from build123d import *

# Parameters (mm, degrees)
SKETCH1_W               = 210
SKETCH1_H               = 80
SKETCH1_R               = 1.5
SKETCH1_R_2             = 9.5
SKETCH1_W_2             = 20
SKETCH1_H_2             = 20
BOSS_EXTRUDE1_DEPTH     = 3
FILLET1_R               = 5
F_1_4_20_TAPPED_HOLE1_D = 5.1054


with BuildPart() as part:
    # Sketch1 → Boss-Extrude1 (new body)
    with BuildSketch(Plane(origin=(0, 0, 0), x_dir=(1, 0, 0), z_dir=(0, 1, 0))):
        with Locations((105, 40)):
            Rectangle(SKETCH1_W, SKETCH1_H)
        with Locations(Location((52.5, 52.5, 0), (0, 0, 270))):
            Circle(SKETCH1_R, mode=Mode.SUBTRACT)
        with Locations(Location((65, 40, 0), (0, 0, 270))):
            Circle(SKETCH1_R, mode=Mode.SUBTRACT)
        with Locations(Location((52.5, 27.5, 0), (0, 0, 270))):
            Circle(SKETCH1_R, mode=Mode.SUBTRACT)
        with Locations(Location((40, 40, 0), (0, 0, 270))):
            Circle(SKETCH1_R, mode=Mode.SUBTRACT)
        with Locations(Location((157.5, 52.5, 0), (0, 0, 270))):
            Circle(SKETCH1_R, mode=Mode.SUBTRACT)
        with Locations(Location((170, 40, 0), (0, 0, 270))):
            Circle(SKETCH1_R, mode=Mode.SUBTRACT)
        with Locations(Location((157.5, 27.5, 0), (0, 0, 270))):
            Circle(SKETCH1_R, mode=Mode.SUBTRACT)
        with Locations(Location((145, 40, 0), (0, 0, 270))):
            Circle(SKETCH1_R, mode=Mode.SUBTRACT)
        with Locations(Location((52.5, 40, 0), (0, 0, 270))):
            Circle(SKETCH1_R_2, mode=Mode.SUBTRACT)
        with Locations(Location((157.5, 40, 0), (0, 0, 270))):
            Circle(SKETCH1_R_2, mode=Mode.SUBTRACT)
        with Locations((105, 40)):
            Rectangle(SKETCH1_W_2, SKETCH1_H_2, mode=Mode.SUBTRACT)
    extrude(amount=-BOSS_EXTRUDE1_DEPTH)

    # Fillet1
    fillet1_edges = [part.edges().sort_by_distance(p)[0] for p in [
        (0, -1.5, -80),
        (210, -1.5, -80),
        (210, -1.5, 0),
        (0, -1.5, 0),
    ]]
    fillet(fillet1_edges, radius=FILLET1_R)

    # 1/4-20 Tapped Hole1 (through all)
    with Locations(Plane(origin=(0, 0, 0), x_dir=(1, 0, 0), z_dir=(0, 1, 0))):
        with Locations((5, 75), (5, 5), (205, 5), (205, 75)):
            Hole(F_1_4_20_TAPPED_HOLE1_D / 2)


solid = part.part
Can you work these out from the model? Positions are in its coordinate system, mm. Give positions to 0.01 mm unless a question says otherwise; leave off trailing zeros. Loops run counter-clockwise (first coordinate to the right, second up) from the corner with the lowest first, then second, coordinate; pieces in that order, holes last. Notation, with made-up numbers: (5, 24) -> (33, 24) arc R20 cw to (33, 52) -> close; hole circle Ø5 at (61.5, 22). An arc over 180 degrees is marked (long way). Return JSON: item names as keys, results as strings.
Q1. We'd pull the mould along X, two halves only. Please class faces 1 (the face through (104, 0, -58)), 2 (the face through (208, -2, -1)), 3 (the face through (207.55, -1.52, -5.11)): released by +X, released by -X, zero draft, split by the parting line, or undercut.
Checks:
{"face 1": "zero draft", "face 2": "released by +X", "face 3": "undercut"}
Q2. I need wall thicknesses on probe 1 along X at (y, z) = (-1.15, -75); probe 2 along Z at (x, y) = (5, -2.25); probe 3 along X at (y, z) = (-0.55, -6). Which ranges of each line are inside material? Lowest first, please.
Checks:
{"probe 1": "x = 0 to 2.45, 7.55 to 202.45, 207.55 to 210", "probe 2": "z = -80 to -77.55, -72.45 to -7.55, -2.45 to 0", "probe 3": "x = 0 to 2.65, 7.35 to 202.65, 207.35 to 210"}
Q3. I want a section at A-A, the plane y = -0.75. Count the separate pieces of the cut face and the enclosed holes in it, then the cut area to 3 significant figures.
Checks:
{"separate pieces": "1", "enclosed holes": "15", "area": "15,700 mm2"}
Q4. I want a section at B-B, the plane x = 162. List the corners of the cut face in (y, z) for me, then the cut area to 3 significant figures.
Checks:
{"outline": "(-3, -80) -> (0, -80) -> (0, -48.37) -> (-3, -48.37) -> close; (-3, -31.63) -> (0, -31.63) -> (0, 0) -> (-3, 0) -> close", "area": "190 mm2"}
Q5. For pin 1 Ø2.5 at (x, z) = (40, -40) entering from +Y; pin 2 Ø3.5 at (x, z) = (157.5, -27.5) entering from +Y, each with a flat end and sliding along its axis, tell me the tip position at first contact or that it passes through.
Checks:
{"pin 1": "passes through", "pin 2": "stops at y = 0"}
